```python
from build123d import *

# Parameters (mm, degrees)
SKETCH1_R               = 12.7
BOSS_EXTRUDE1_DEPTH     = 203.2
SKETCH2_R               = 9.525
BOSS_EXTRUDE2_DEPTH     = 7.62
CHAMFER1_SIZE           = 0.635
SKETCH4_W               = 7.62
SKETCH4_H               = 42.672
CUT_EXTRUDE1_DEPTH      = 25.4
CUT_EXTRUDE1_DEPTH_BACK = 25.4
SKETCH5_R               = 3.175
CUT_EXTRUDE2_DEPTH      = 25.4


with BuildPart() as part:
    # Sketch1 → Boss-Extrude1 (new body)
    with BuildSketch(Plane(origin=(0, 0, 0), x_dir=(1, 0, 0), z_dir=(0, 1, 0))):
        Circle(SKETCH1_R)
    extrude(amount=BOSS_EXTRUDE1_DEPTH)

    # Sketch2 → Boss-Extrude2 (add)
    with BuildSketch(Plane(origin=(0, 0, 0), x_dir=(-1, 0, 0), z_dir=(0, -1, 0))):
        Circle(SKETCH2_R)
    extrude(amount=BOSS_EXTRUDE2_DEPTH)

    # Chamfer1
    chamfer1_edges = [part.edges().sort_by_distance(p)[0] for p in [
        (-12.7, 0, 0),
        (9.525, -7.62, 0),
    ]]
    chamfer(chamfer1_edges, length=CHAMFER1_SIZE)

    # Sketch4 → Cut-Extrude1 (cut, two sides)
    with BuildSketch(Plane(origin=(0, 0, 0), x_dir=(0, 0, -1), z_dir=(1, 0, 0))) as cut_extrude1_sk:
        with Locations((-8.89, 115.316)):
            Rectangle(SKETCH4_W, SKETCH4_H)
    extrude(amount=CUT_EXTRUDE1_DEPTH, mode=Mode.SUBTRACT)
    extrude(cut_extrude1_sk.sketch, amount=-CUT_EXTRUDE1_DEPTH_BACK, mode=Mode.SUBTRACT)

    # Sketch5 → Cut-Extrude2 (cut)
    with BuildSketch(Plane.XY.offset(5.08)):
        with Locations((0, 104.902)):
            Circle(SKETCH5_R)
        with Locations((0, 127)):
            Circle(SKETCH5_R)
    extrude(amount=-CUT_EXTRUDE2_DEPTH, mode=Mode.SUBTRACT)


solid = part.part
```
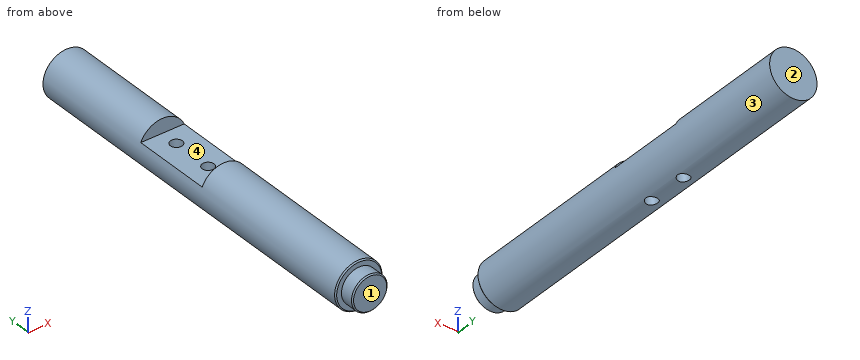
Input: part model. Units: mm. Frame: model coordinates. Face numbers are marked on the shaded views. Give positions to 0.01 mm unless a question says otherwise; leave off trailing zeros. Order: outer loops, then holes, each group sorted by start corner. A loop starts at its lowest first (then second) coordinate and runs counter-clockwise, first axis right, second up. Notation, with made-up numbers: M 37.5,69.5 L 54.5,69.5 A30 ccw 54.5,108.5 Z; hole C 88.5,-10 d2. An arc over 180 degrees is marked long. One line per question, with ' | ' between items.
1) Contact query for flat-ended pins moving along their axis: P1, Ø4, axis at x = 0, y = 104.902, coming from the -Z side; P2, Ø1.5, axis at y = 130.5, z = 4, coming from the -X side; P3, Ø2, axis at x = -2.5, y = 35, coming from the +Z side; P4, Ø10, axis at x = 0, y = 127, coming from the +Z side. Output: stop coordinate, or through.
Filled in:
P1: passes through | P2: stops at x = -12.28 | P3: stops at z = 12.61 | P4: stops at z = 5.08
2) Draft query along Y for the marked faces 1, 2, 3 and 4. Return one class per face: pulls with the +Y half, pulls with the -Y half, needs draft (parallel to the pull), parting line crosses it, or undercut.
Filled in:
face 1: pulls with the -Y half | face 2: pulls with the +Y half | face 3: needs draft | face 4: undercut
3) Section D-D on y = 127. Output: boundary loops of the cut face in (x, z) (3 decimals), and give its area (3 significant figures).
Filled in:
outline: M -11.64,5.08 A12.7 ccw -3.175,-12.297 L -3.175,5.08 Z; M 3.175,-12.297 A12.7 ccw 11.64,5.08 L 3.175,5.08 Z | area: 267 mm2
4) Ray query, L1, parallel to Y at x = 0, z = 0 (3 decimals); L2, parallel to Y at x = -1.25, z = 9.5; L3, parallel to Y at x = 11, z = 1. Return the intervals inside material, ascending.
Filled in:
L1: y = -7.62 to 101.727, 108.077 to 123.825, 130.175 to 203.2 | L2: y = 0 to 93.98, 136.65 to 203.2 | L3: y = 0 to 203.2
5) Section A-A on x = 0. Output: boundary loops of the cut face in (y, z) (3 decimals), and give its area (3 significant figures).
Filled in:
outline: M -7.62,-8.89 L -6.985,-9.525 L 0,-9.525 L 0,-12.065 L 0.635,-12.7 L 101.727,-12.7 L 101.727,5.08 L 93.98,5.08 L 93.98,12.7 L 0.635,12.7 L 0,12.065 L 0,9.525 L -6.985,9.525 L -7.62,8.89 Z; M 108.077,-12.7 L 123.825,-12.7 L 123.825,5.08 L 108.077,5.08 Z; M 130.175,-12.7 L 203.2,-12.7 L 203.2,12.7 L 136.652,12.7 L 136.652,5.08 L 130.175,5.08 Z | area: 4,750 mm2
6) Section B-B on z = 0. Output: boundary loops of the cut face in (x, y) (3 decimals).
Filled in:
outline: M -12.7,0.635 L -12.065,0 L -9.525,0 L -9.525,-6.985 L -8.89,-7.62 L 8.89,-7.62 L 9.525,-6.985 L 9.525,0 L 12.065,0 L 12.7,0.635 L 12.7,203.2 L -12.7,203.2 Z; hole C 0,104.902 d6.35; hole C 0,127 d6.35
7) Section C-C on y = 184.5. Output: boundary loops of the cut face in (x, z).
Filled in:
outline: C 0,0 d25.4
